Input: part model. Units: mm. Frame: model coordinates. A direction names the side the tool comes from. Give positions to 0.01 mm unless a question says otherwise; leave off trailing zeros. Write each loop counter-clockwise with the first axis right and the second up, starting at its lowest first coordinate (ties: lowest second). Pieces come first, ordered by that corner, then holes. Notation, with made-up numbers: (34, 83) -> (86, 83) arc R19 cw to (86, 94) -> close; hole circle Ø5 at (-7.75, -39). An arc over 180 degrees is marked (long way). Answer as a JSON object with one key per item and string values. Group by question number.
from build123d import *

# Parameters (mm, degrees)
F0_W     = 135.89
F0_H     = 75.946
F0_R     = 1.651
F1_DEPTH = 2.794
F3_R     = 1.2319
F4_DEPTH = 2.795
F5_R     = 3.656552
F5_R_2   = 1.2319
F6_DEPTH = 6.35
F7_R     = 6.19125
F7_R_2   = 3.90525
F8_DEPTH = 9.145


with BuildPart() as f1:
    # F0 (on Top) → F1 (new body)
    with BuildSketch(Plane.XY):
        with Locations((67.945, 37.973)):
            Rectangle(F0_W, F0_H)
        with Locations((13.81125, 3.6068)):
            Circle(F0_R, mode=Mode.SUBTRACT)
        with Locations((122.07875, 3.6068)):
            Circle(F0_R, mode=Mode.SUBTRACT)
        with BuildLine():
            ThreePointArc((100.087966, 61.7855), (111.135553, 54.848267), (117.1575, 43.276296))
            Line((117.1575, 43.276296), (117.1575, 32.669704))
            ThreePointArc((117.1575, 32.669704), (111.135553, 21.097733), (100.087966, 14.1605))
            Line((100.087966, 14.1605), (85.586034, 14.1605))
            ThreePointArc((85.586034, 14.1605), (75.803192, 19.821938), (69.5325, 29.225889))
            Line((69.5325, 29.225889), (69.5325, 46.720111))
            ThreePointArc((69.5325, 46.720111), (75.803192, 56.124062), (85.586034, 61.7855))
            Line((85.586034, 61.7855), (100.087966, 61.7855))
        make_face(mode=Mode.SUBTRACT)
        with BuildLine():
            ThreePointArc((18.7325, 43.276296), (24.754447, 54.848267), (35.802034, 61.7855))
            Line((35.802034, 61.7855), (50.303966, 61.7855))
            ThreePointArc((50.303966, 61.7855), (60.086808, 56.124062), (66.3575, 46.720111))
            Line((66.3575, 46.720111), (66.3575, 29.225889))
            ThreePointArc((66.3575, 29.225889), (60.086808, 19.821938), (50.303966, 14.1605))
            Line((50.303966, 14.1605), (35.802034, 14.1605))
            ThreePointArc((35.802034, 14.1605), (24.754447, 21.097733), (18.7325, 32.669704))
            Line((18.7325, 32.669704), (18.7325, 43.276296))
        make_face(mode=Mode.SUBTRACT)
        with Locations((13.81125, 72.3392)):
            Circle(F0_R, mode=Mode.SUBTRACT)
        with Locations((122.07875, 72.3392)):
            Circle(F0_R, mode=Mode.SUBTRACT)
    extrude(amount=F1_DEPTH)

    # F3 (on face) → F4 (cut, through all)
    with BuildSketch(Plane.XY.offset(2.794)):
        with Locations((22.7711, 58.0644)):
            Circle(F3_R)
        with Locations((62.9539, 58.0644)):
            Circle(F3_R)
        with Locations((72.9361, 58.0644)):
            Circle(F3_R)
        with Locations((113.1189, 58.0644)):
            Circle(F3_R)
        with Locations((113.1189, 17.8816)):
            Circle(F3_R)
        with Locations((72.9361, 17.8816)):
            Circle(F3_R)
        with Locations((62.9539, 17.8816)):
            Circle(F3_R)
        with Locations((22.7711, 17.8816)):
            Circle(F3_R)
    extrude(amount=-F4_DEPTH, mode=Mode.SUBTRACT)

    # F5 (on face) → F6 (join)
    with BuildSketch(Plane.XY.offset(2.794)):
        with Locations((22.7711, 58.0644)):
            Circle(F5_R)
        with Locations((22.7711, 58.0644)):
            Circle(F5_R_2, mode=Mode.SUBTRACT)
        with Locations((62.9539, 58.0644)):
            Circle(F5_R)
        with Locations((62.9539, 58.0644)):
            Circle(F5_R_2, mode=Mode.SUBTRACT)
        with Locations((72.9361, 58.0644)):
            Circle(F5_R)
        with Locations((72.9361, 58.0644)):
            Circle(F5_R_2, mode=Mode.SUBTRACT)
        with Locations((113.1189, 58.0644)):
            Circle(F5_R)
        with Locations((113.1189, 58.0644)):
            Circle(F5_R_2, mode=Mode.SUBTRACT)
        with Locations((113.1189, 17.8816)):
            Circle(F5_R)
        with Locations((113.1189, 17.8816)):
            Circle(F5_R_2, mode=Mode.SUBTRACT)
        with Locations((72.9361, 17.8816)):
            Circle(F5_R)
        with Locations((72.9361, 17.8816)):
            Circle(F5_R_2, mode=Mode.SUBTRACT)
        with Locations((62.9539, 17.8816)):
            Circle(F5_R)
        with Locations((62.9539, 17.8816)):
            Circle(F5_R_2, mode=Mode.SUBTRACT)
        with Locations((22.7711, 17.8816)):
            Circle(F5_R)
        with Locations((22.7711, 17.8816)):
            Circle(F5_R_2, mode=Mode.SUBTRACT)
    extrude(amount=F6_DEPTH)

    # F7 (on face) → F8 (cut, through all)
    with BuildSketch(Plane(origin=(0, 0, 0), x_dir=(1, 0, 0), z_dir=(0, 0, -1))):
        with Locations((9.36625, -62.258438)):
            Circle(F7_R)
        with Locations((9.36625, -46.068146)):
            Circle(F7_R)
        with Locations((21.82186, -68.86575)):
            Circle(F7_R_2)
        with Locations((34.9999, -68.86575)):
            Circle(F7_R_2)
        with Locations((48.17794, -68.86575)):
            Circle(F7_R_2)
        with Locations((61.35598, -68.86575)):
            Circle(F7_R_2)
        with Locations((126.52375, -46.068146)):
            Circle(F7_R)
        with Locations((126.52375, -62.258438)):
            Circle(F7_R)
        with Locations((74.53402, -68.86575)):
            Circle(F7_R_2)
        with Locations((87.71206, -68.86575)):
            Circle(F7_R_2)
        with Locations((100.8901, -68.86575)):
            Circle(F7_R_2)
        with Locations((114.06814, -68.86575)):
            Circle(F7_R_2)
        with Locations((126.52375, -29.877854)):
            Circle(F7_R)
        with Locations((126.52375, -13.687562)):
            Circle(F7_R)
        with Locations((114.06814, -7.08025)):
            Circle(F7_R_2)
        with Locations((100.8901, -7.08025)):
            Circle(F7_R_2)
        with Locations((87.71206, -7.08025)):
            Circle(F7_R_2)
        with Locations((74.53402, -7.08025)):
            Circle(F7_R_2)
        with Locations((61.35598, -7.08025)):
            Circle(F7_R_2)
        with Locations((48.17794, -7.08025)):
            Circle(F7_R_2)
        with Locations((34.9999, -7.08025)):
            Circle(F7_R_2)
        with Locations((21.82186, -7.08025)):
            Circle(F7_R_2)
        with Locations((9.36625, -13.687562)):
            Circle(F7_R)
        with Locations((9.36625, -29.877854)):
            Circle(F7_R)
    extrude(amount=-F8_DEPTH, mode=Mode.SUBTRACT)


solid = f1.part
1. Mould query, pull axis Y, two halves, no side actions, for faces 4 (the face through (67, 0, 1)), 5 (the face through (70.034, 55.839, 5.925)), 6 (the face through (23, 56, 9.144)). Classes: pulls with the +Y half, pulls with the -Y half, needs draft (parallel to the pull), parting line crosses it, or undercut.
2. Section B-B (y = 37.5). Return the cut outline in (x, z), plus the area to 3 significant figures.
3. Section A-A (z = 4.25). State how many separate pieces and enclosed holes the cut face has, plus the area to 3 significant figures.
4. Reachability of faces 1 (the face through (67, 75.946, 1)), 2 (the face through (20.076, 20.353, 5.925)), 3 (the face through (69.532, 38, 1)) from +Z, -Z, +X, -X, +Y, -Y: full face, straight path, thin tool, end or side. Return the list, or none.
5. Line query: line 1 (Y direction, x = 61.5, z = 2.5); line 2 (X direction, y = 51.5, z = 0.5); line 3 (Y direction, x = 100, z = 1.25). Output: solid intervals per line, ascending.
6. Contact query for flat-ended pins moving along their axis: pin 1 Ø9 at (x, y) = (48.18, 68.87) entering from +Z; pin 2 Ø4 at (y, z) = (57.5, 5.5) entering from -X; pin 3 Ø2 at (x, y) = (62.95, 58.06) entering from -Z. Output: stop coordinate, or through.
Working result:
{
 "1": {"face 4": "pulls with the -Y half", "face 5": "undercut", "face 6": "needs draft"},
 "2": {"outline": "(0, 0) -> (18.73, 0) -> (18.73, 2.79) -> (0, 2.79) -> close; (66.36, 0) -> (69.53, 0) -> (69.53, 2.79) -> (66.36, 2.79) -> close; (117.16, 0) -> (135.89, 0) -> (135.89, 2.79) -> (117.16, 2.79) -> close", "area": "114 mm^2"},
 "3": {"separate pieces": "8", "enclosed holes": "8", "area": "298 mm^2"},
 "4": {"face 1": "+Z, -Z, +X, -X, +Y", "face 2": "+Z", "face 3": "+Z, -Z"},
 "5": {"line 1": "y = 0 to 3.18, 10.98 to 21.26, 54.69 to 64.96, 72.77 to 75.95", "line 2": "x = 0 to 6.4, 12.34 to 22.16, 63.95 to 71.94, 113.73 to 123.55, 129.49 to 135.89", "line 3": "y = 0 to 3.28, 10.88 to 14.16, 61.79 to 65.06, 72.67 to 75.95"},
 "6": {"pin 1": "stops at z = 2.79", "pin 2": "stops at x = 19.11", "pin 3": "passes through"}
}
